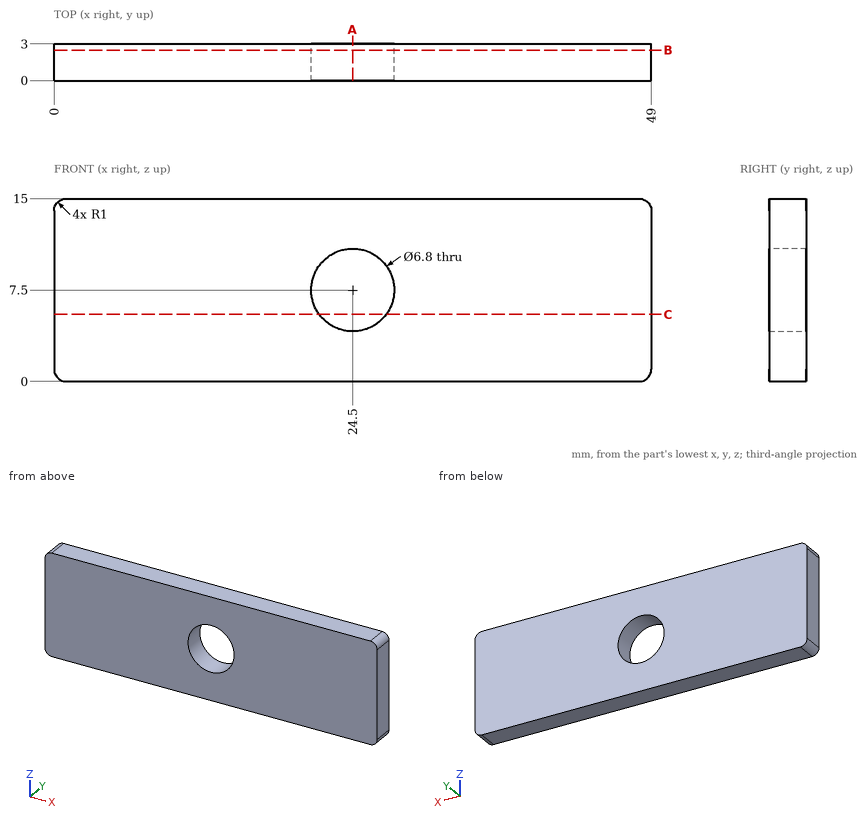
Part print with two shaded views. Sizes in mm from the minimum x, y, z corner. Round coordinates to 2 decimals unless told otherwise and drop trailing zeros. Loops run counter-clockwise (first coordinate to the right, second up) from the corner with the lowest first, then second, coordinate; pieces in that order, holes last. Notation, with made-up numbers: M 31.5,85.5 L 41.5,85.5 A25 cw 41.5,116.5 Z; hole C 71.25,47 d9. An arc over 180 degrees is marked long. Put each result on its own line as item: value. Start each with the question number.
Item 1: Drill centre lines: line 1 along X through (y, z) = (1.9, 7.5); line 2 along X through (y, z) = (2.3, 6.5); line 3 along Z through (x, y) = (23.5, 0.65). Where is each one in solid material? Low to high.
Item 2: Cut at A-A (x = 24.5). List the corners of the cut face in (y, z).
Item 3: Cut at B-B (y = 2.5). List the corners of the cut face in (x, z), then the cut area to 3 significant figures.
Item 4: Cut at C-C (z = 5.5). List the corners of the cut face in (x, y), then the cut area to 3 significant figures.
Item 5: Drop flat-ended pins along their axis: P1, Ø1, axis at y = 0.5, z = 2.5, coming from the -X side; P2, Ø5.5, axis at x = 24.5, z = 7.5, coming from the +Y side. Give the stop position or say it passes through.
Answer block:
1. line 1: 0 to 21.1, 27.9 to 49
1. line 2: 0 to 21.25, 27.75 to 49
1. line 3: 0 to 4.25, 10.75 to 15
2. outline: M 0,0 L 3,0 L 3,4.1 L 0,4.1 Z; M 0,10.9 L 3,10.9 L 3,15 L 0,15 Z
3. outline: M 0,1 A1 ccw 1,0 L 48,0 A1 ccw 49,1 L 49,14 A1 ccw 48,15 L 1,15 A1 ccw 0,14 Z; hole C 24.5,7.5 d6.8
3. area: 698 mm2
4. outline: M 0,0 L 21.75,0 L 21.75,3 L 0,3 Z; M 27.25,0 L 49,0 L 49,3 L 27.25,3 Z
4. area: 131 mm2
5. P1: x = 0
5. P2: through
